Autodesk Fusion 360 part; units mm, degrees
sketch "Sketch1" plane through (0, 0, 0) normal (0, 0, 1) x (1, 0, 0)
  line L0 (65, -48.5) -> (-65, -48.5)
  line L1 (-65, -48.5) -> (-65, 48.5)
  line L2 (-65, 48.5) -> (65, 48.5)
  line L3 (65, 48.5) -> (65, -48.5)
  line L4 (65, -48.5) -> (-65, 48.5) construction
  line L5 (-65, -48.5) -> (65, 48.5) construction
  line L6 (-65, 48.5) -> (2983, 48.5)
  line L7 (2983, 48.5) -> (2983, -49)
  line L8 (2983, -49) -> (-65, -49)
  line L9 (-65, -49) -> (-65, 48.5)
  line L10 (-65, 48.5) -> (-55, 48.5)
  line L11 (-55, 48.5) -> (-55, -49)
  line L12 (-55, -49) -> (-65, -49)
  line L13 (-65, -49) -> (-65, 48.5)
  line L14 (65, 48.5) -> (59, 48.5)
  line L15 (59, 48.5) -> (59, 38.5)
  line L16 (59, 38.5) -> (65, 38.5)
  line L17 (65, 38.5) -> (65, 48.5)
  line L18 (59, 38.5) -> (59, -49)
  line L19 (-65, 48.5) -> (59, 48.5)
  line L20 (59, 48.5) -> (59, 47.5)
  line L21 (59, 47.5) -> (-65, 47.5)
  line L22 (-65, 47.5) -> (-65, 48.5)
  line L23 (-65, -49) -> (65, -49)
  line L24 (65, -49) -> (65, -48)
  line L25 (65, -48) -> (-65, -48)
  line L26 (-65, -48) -> (-65, -49)
  line L27 (-56, 38) -> (-65, 38)
  line L28 (-65, 38) -> (-65, 23)
  line L29 (-65, 23) -> (-56, 23)
  line L30 (-56, 23) -> (-56, 38)
  line L31 (-56, -41) -> (-65, -41)
  line L32 (-65, -41) -> (-65, 14)
  line L33 (-65, 14) -> (-56, 14)
  line L34 (-56, 14) -> (-56, -41)
  line L35 (-65, 48.5) -> (-60, 48.5) construction
  line L36 (-60, 48.5) -> (-60, 43.5) construction
  circle A0 centre (-60, 43.5) radius 1.5
  line L37 (65, 48.5) -> (53, 48.5) construction
  line L38 (53, 48.5) -> (53, 41.5) construction
  circle A1 centre (53, 41.5) radius 1.5
  line L39 (65.5, 45) -> (62, 45)
  line L40 (65.5, 42) -> (62, 42)
  arc A2 (62, 45) -> (62, 42) centre (62, 43.5) ccw
  line L41 (-65, 48.5) -> (12.5, 48.5) construction
  line L42 (12.5, 48.5) -> (12.5, 18.5) construction
  line L43 (12.5, 18.5) -> (12.5, -14.5) construction
  circle A3 centre (12.5, 18.5) radius 1.5
  circle A4 centre (12.5, -14.5) radius 1.5
  line L44 (-65, -48.5) -> (-60, -48.5) construction
  line L45 (-60, -48.5) -> (-60, -43.5) construction
  circle A5 centre (-60, -43.5) radius 1.5
  dimension "d1" = 130
  dimension "d2" = 97
  dimension "d3" = 3048
  dimension "d4" = 10
  dimension "d5" = 6
  dimension "d6" = 10
  dimension "d7" = 1
  dimension "d8" = 1
  dimension "d9" = 15
  dimension "d10" = 55
  dimension "d11" = 5
  dimension "d12" = 5
  dimension "d13" = 3
  dimension "d14" = 12
  dimension "d15" = 7
  dimension "d16" = 3
  dimension "d17" = 77.5
  dimension "d18" = 30
  dimension "d19" = 33
  dimension "d20" = 3
  dimension "d21" = 3
  dimension "d22" = 5
  dimension "d23" = 5
  dimension "d24" = 3
extrude "Extrude1" add sketch "Sketch1" along normal blind 50 contours L0 L3 L18 L24 L25 | L0 L11 L18 L25 | L0 L1 L9 L11 L13 L25 L26 | L11 L15 L18 L21 L25 | L1 L2 L6 L9 L10 L11 L13 L19 L21 L22 | L2 L6 L11 L15 L19 L20 L21 | A1 | A3 | A4 makes body 1
extrude "Extrude2" add sketch "Sketch1" along normal blind 20 separate body contours L1 L9 L13 L31 L32 L33 L34 | L1 L9 L13 L27 L28 L29 L30 makes body 2 at (-65, -22.6667, 6.6667) makes body 3 at (-56, 28, 6.6667)
extrude "Extrude3" add sketch "Sketch1" along normal blind 1 contours L3 L16 L18 L25 | L2 L3 L6 L14 L15 L16 L17 L20 L39 L40 A2 | L1 L9 L11 L13 L21 L25 L27 L29 L30 L31 L33 L34 bodies 1 2 3
extrude "Extrude4" cut sketch "Sketch1" along normal blind 5 contours A1 | A3 | A4 bodies 1
sketch "Sketch2" plane through (0, -48.5, 0) normal (0, -1, 0) x (1, 0, 0)
  line L0 (-65, 0) -> (65, 0)
  line L1 (65, 0) -> (65, 50)
  line L2 (65, 50) -> (-65, 50)
  line L3 (-65, 50) -> (-65, 0)
  line L4 (-65, 50) -> (65, 50)
  line L5 (-65, 0) -> (-65, 50)
  line L6 (65, 0) -> (-65, 0)
  line L7 (65, 0) -> (65, 50)
  line L8 (-65, 50) -> (-59, 50) construction
  line L9 (-59, 50) -> (-59, 42) construction
  circle A0 centre (-59, 42) radius 1.5
  line L10 (65, 50) -> (65, 40) construction
  line L11 (65, 38) -> (62, 38)
  line L12 (65, 42) -> (62, 42)
  arc A1 (62, 42) -> (62, 38) centre (62, 40) ccw
  line L13 (-65, 50) -> (-32.5, 50) construction
  line L14 (-32.5, 50) -> (-32.5, 30) construction
  line L15 (65, 50) -> (44, 50) construction
  line L16 (44, 50) -> (44, 40) construction
  line L17 (44, 40) -> (44, 21) construction
  circle A2 centre (-32.5, 30) radius 1.5
  circle A3 centre (44, 40) radius 1.5
  circle A4 centre (44, 21) radius 1.5
  dimension "d33" = 6
  dimension "d34" = 8
  dimension "d35" = 3
  dimension "d36" = 10
  dimension "d37" = 32.5
  dimension "d38" = 20
  dimension "d39" = 21
  dimension "d40" = 10
  dimension "d41" = 19
  dimension "d42" = 3
  dimension "d43" = 3
  dimension "d44" = 3
extrude "Extrude5" cut sketch "Sketch2" against normal blind 5 contours L1 L7 L11 L12 A1 | A0 | A2 | A3 | A4 bodies 1
equation "d3 = 10'-0\""
Geometry check sheet. Reference: the model listing, model coordinates, mm. A direction names the side the tool comes from. Round coordinates to 2 decimals unless told otherwise and drop trailing zeros. Order: outer loops, then holes, each group sorted by start corner. A loop starts at its lowest first (then second) coordinate and runs counter-clockwise, first axis right, second up. Notation, with made-up numbers: (47, -12.75) -> (59, -12.75) arc R29 ccw to (59, 26.25) -> close; hole circle Ø9 at (-21.5, -27.5). An arc over 180 degrees is marked (long way). Return JSON: item names as keys, results as strings. Group by question number.
Q1. Material ranges on probe 1 along X at (y, z) = (-8.5, 5); probe 2 along X at (y, z) = (14.5, 14), recorded low to high. Write a range as from..to.
Q2. Release check for a two-part mould opening along Z. For faces 5 (the flat face through (44, -43.5, 21)), 6 (the flat face through (-60, 47.5, 25)), 7 (the flat face through (14, 1, 50)) record: released by +Z, released by -Z, zero draft, split by the parting line, or undercut.
Q3. Section check C-C, the plane z = 26. Record the boundary of the cut face in (x, y), plus the area to 3 significant figures.
Q4. Tool access check on faces 1 (the flat face through (59, 1, 25)), 2 (the flat face through (44, -43.5, 40)), 3 (the flat face through (-56, 30, 10)), 4 (the flat face through (12, -14, 5)). Record the directions out of +Z, -Z, +X, -X, +Y, -Y that give a thin tool (end or side, any length) a straight path to the whole face; none if there is none.
Q5. Gauge pin test, flat ends, axial feed: pin 1 (1.5 mm diameter, centred on x = 44, z = 40, fed in from -Y); pin 2 (2.5 mm diameter, centred on x = 12.5, y = -14.5, fed in from -Z); pin 3 (2.5 mm diameter, centred on x = -60, y = -43.5, fed in from +Z); pin 4 (16.5 mm diameter, centred on y = 30.5, z = 11.5, fed in from +X). Record the tip position at first contact, or that the pin passes through.
Q6. Section check A-A, the plane z = 18. Record the boundary of the cut face in (x, y), plus the area to 3 significant figures.
Q7. Section check B-B, the plane y = -30. Record the boundary of the cut face in (x, z), plus the area to 3 significant figures.
Numbers:
{
 "1": {"probe 1": "-65..-56, -55..59", "probe 2": "-55..59"},
 "2": {"face 5": "undercut", "face 6": "zero draft", "face 7": "released by +Z"},
 "3": {"outline": "(-65, -48.5) -> (65, -48.5) -> (65, -48) -> (59, -48) -> (59, 48.5) -> (-65, 48.5) -> (-65, 47.5) -> (-55, 47.5) -> (-55, -48) -> (-65, -48) -> close", "area": "11,100 mm^2"},
 "4": {"face 1": "+Z, +X, +Y", "face 2": "-Y", "face 3": "+Z", "face 4": "-Z"},
 "5": {"pin 1": "y = -43.5", "pin 2": "z = 5", "pin 3": "through", "pin 4": "x = 59"},
 "6": {"outline": "(-65, -48.5) -> (65, -48.5) -> (65, -48) -> (59, -48) -> (59, 48.5) -> (-65, 48.5) -> (-65, 47.5) -> (-55, 47.5) -> (-55, -48) -> (-65, -48) -> close; (-65, -41) -> (-56, -41) -> (-56, 14) -> (-65, 14) -> close; (-65, 23) -> (-56, 23) -> (-56, 38) -> (-65, 38) -> close", "area": "11,700 mm^2"},
 "7": {"outline": "(-65, 0) -> (65, 0) -> (65, 1) -> (59, 1) -> (59, 50) -> (-55, 50) -> (-55, 1) -> (-56, 1) -> (-56, 20) -> (-65, 20) -> close", "area": "5,890 mm^2"}
}
